Design review of the part shown in the three views and the two pictorial views. Dimensions are in mm from the part's minimum x, y and z. A direction names the side the tool comes from. Round coordinates to 2 decimals unless told otherwise and drop trailing zeros. Order: outer loops, then holes, each group sorted by start corner. A loop starts at its lowest first (then second) coordinate and runs counter-clockwise, first axis right, second up. Notation, with made-up numbers: (11, -14) - (39, -14) arc R22 ccw to (39, 14) - close; hole circle Ø3 at (-37.5, 24). An arc over 180 degrees is marked (long way). One line per question, with ' | ' between items. Start each with the question number.
Item 1: Tool access review of the marked faces 1 and 2: name each direction out of +Z, -Z, +X, -X, +Y, -Y from which nothing blocks a thin tool from reaching the whole face with its end or side.
Item 2: Add section D-D on z = 10. State the section outline as (x, y) points, and give its area (3 significant figures).
Item 3: Add section B-B on x = 20. State the section outline as (y, z) points, and give its area (3 significant figures).
Item 4: Add section A-A on z = 16.5. State the section outline as (x, y) points, and give its area (3 significant figures).
Item 5: For L1, parallel to Z at x = 31, y = 37.5; L2, parallel to Z at x = 36, y = 35; L3, parallel to Y at x = 18, z = 6, list the stretches that pass through material, from the lowest coordinate up. Write a range as [from, to].
Item 6: Insertion check: pin 1 Ø1.7 at (x, y) = (6, 35) entering from -Z; pin 2 Ø12 at (x, y) = (27.5, 13.5) entering from -Z. Each pin has a flat end and moves straight along its axis. Give the tip position at first contact, or say it passes through.
Item 7: Draft analysis for pull direction Y (two halves, no side actions). For the marked faces 3, 4 and 5, state which applies: +Y half, -Y half, draft (parallel to the pull), parting line (faces both ways), or undercut.
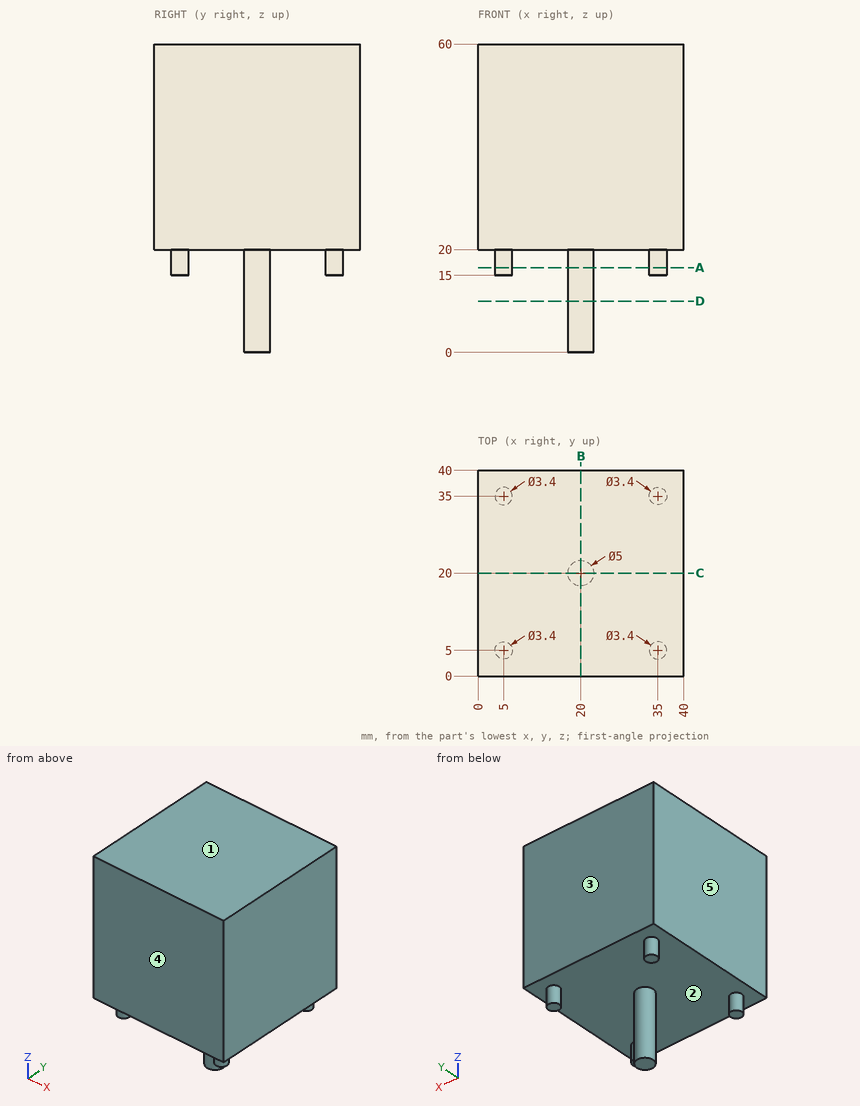
Determined:
1) face 1: +Z, +X, -X, +Y, -Y | face 2: -Z
2) outline: circle Ø5 at (20, 20) | area: 19.6 mm2
3) outline: (0, 20) - (17.5, 20) - (17.5, 0) - (22.5, 0) - (22.5, 20) - (40, 20) - (40, 60) - (0, 60) - close | area: 1,700 mm2
4) outline: circle Ø3.4 at (5, 5); circle Ø3.4 at (5, 35); circle Ø5 at (20, 20); circle Ø3.4 at (35, 5); circle Ø3.4 at (35, 35) | area: 56.0 mm2
5) L1: [20, 60] | L2: [15, 60] | L3: [18.5, 21.5]
6) pin 1: z = 15 | pin 2: z = 20
7) face 3: +Y half | face 4: -Y half | face 5: draft
